The figure shows three views and two pictorial views of one solid part (mm, origin at its lowest corner). Answer the questions. A direction names the side the tool comes from. Give positions to 0.01 mm unless a question says otherwise; leave off trailing zeros. Loops run counter-clockwise (first coordinate to the right, second up) from the corner with the lowest first, then second, coordinate; pieces in that order, holes last. Notation, with made-up numbers: (84.5, 42.25) - (106.5, 42.25) arc R29 cw to (106.5, 79.25) - close; hole circle Ø2 at (-7.75, 13). An arc over 180 degrees is marked (long way). Use a Markdown table: item, result. Add a question column.
Item 1: Which of the six approach directions +Z, -Z, +X, -X, +Y, -Y give full straight-line access (tool end or side, diameter ignored) to the marked faces 5, 6, 7 and 8?
Item 2: A cutting plane is placed at A-A (y = 17). Determine the outline of the cut face in (x, z), plus the area to 3 significant figures.
Item 3: A cutting plane is placed at C-C (z = 18). Determine the outline of the cut face in (x, y).
Item 4: A cutting plane is placed at B-B (z = 29). Determine the outline of the cut face in (x, y).
Item 5: For a pull along Y with two mould halves and no side action, classify the marked faces 1, 2, 3 and 4 as +Y half, -Y half, draft (parallel to the pull), parting line (faces both ways), or undercut.
Item 6: Consider probe 1 along X at (y, z) = (35, 18); probe 2 along Y at (x, z) = (57.5, 33.5); probe 3 along Z at (x, y) = (4, 17). Determine where each line is inside the solid, lowest interval first. Write a range as [from, to].
Item 7: Each of these flat-tipped pins is pushed along its axis until it touches: P1, Ø10, axis at x = 26, y = 16.5, coming from the +Z side; P2, Ø3, axis at x = 59.5, y = 25, coming from the +Z side; P3, Ø5, axis at y = 8.5, z = 16, coming from the -X side. Where does it stop, or does it pass through?
Item 8: A cutting plane is placed at D-D (y = 3.5). Determine the outline of the cut face in (x, z), plus the area to 3 significant figures.
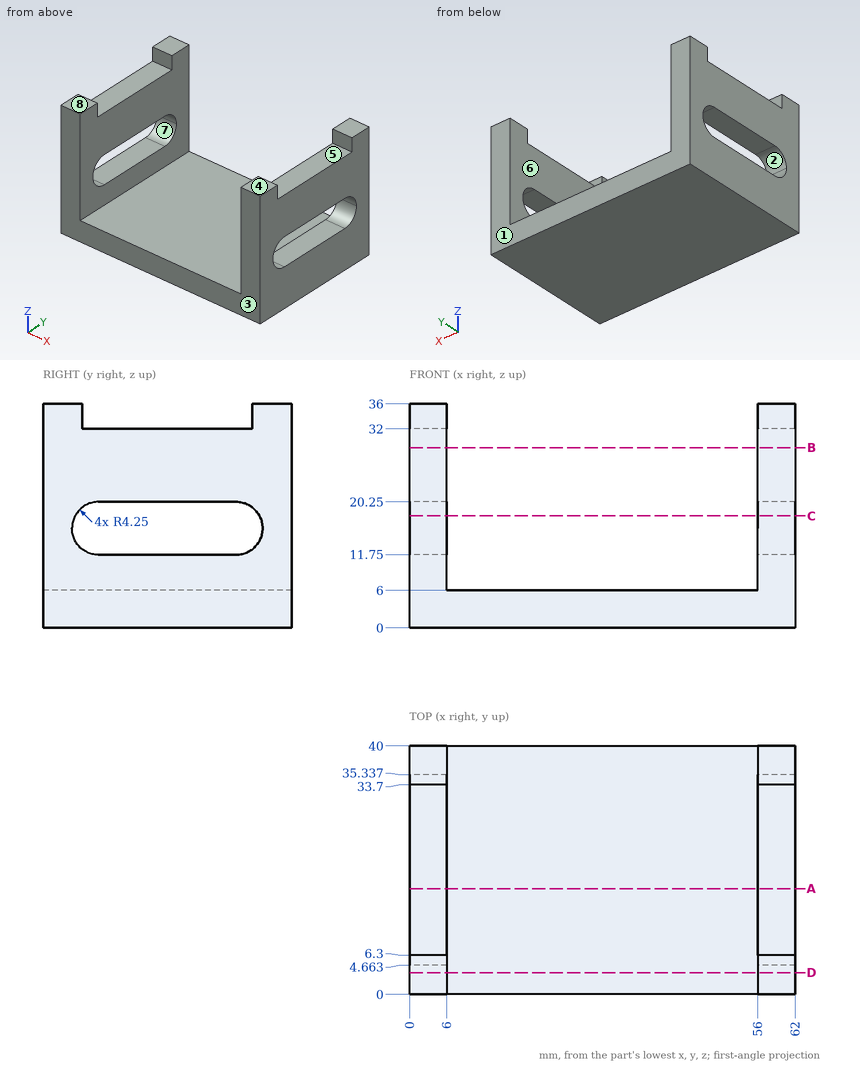
Geometry says:
| question | item | result |
|---|---|---|
| 1 | face 5 | +Z, +X, -X |
| 1 | face 6 | +Z, +Y, -Y |
| 1 | face 7 | +X, -X |
| 1 | face 8 | +Z, +X, -X, +Y, -Y |
| 2 | outline | (0, 0) - (62, 0) - (62, 11.75) - (56, 11.75) - (56, 6) - (6, 6) - (6, 11.75) - (0, 11.75) - close; (0, 20.25) - (6, 20.25) - (6, 32) - (0, 32) - close; (56, 20.25) - (62, 20.25) - (62, 32) - (56, 32) - close |
| 2 | area | 582 mm² |
| 3 | outline | (0, 0) - (6, 0) - (6, 5.16) - (0, 5.16) - close; (0, 34.84) - (6, 34.84) - (6, 40) - (0, 40) - close; (56, 0) - (62, 0) - (62, 5.16) - (56, 5.16) - close; (56, 34.84) - (62, 34.84) - (62, 40) - (56, 40) - close |
| 4 | outline | (0, 0) - (6, 0) - (6, 40) - (0, 40) - close; (56, 0) - (62, 0) - (62, 40) - (56, 40) - close |
| 5 | face 1 | +Y half |
| 5 | face 2 | undercut |
| 5 | face 3 | -Y half |
| 5 | face 4 | draft |
| 6 | probe 1 | [0, 6], [56, 62] |
| 6 | probe 2 | [0, 6.3], [33.7, 40] |
| 6 | probe 3 | [0, 11.75], [20.25, 32] |
| 7 | P1 | z = 6 |
| 7 | P2 | z = 32 |
| 7 | P3 | through |
| 8 | outline | (0, 0) - (62, 0) - (62, 36) - (56, 36) - (56, 6) - (6, 6) - (6, 36) - (0, 36) - close |
| 8 | area | 732 mm² |
